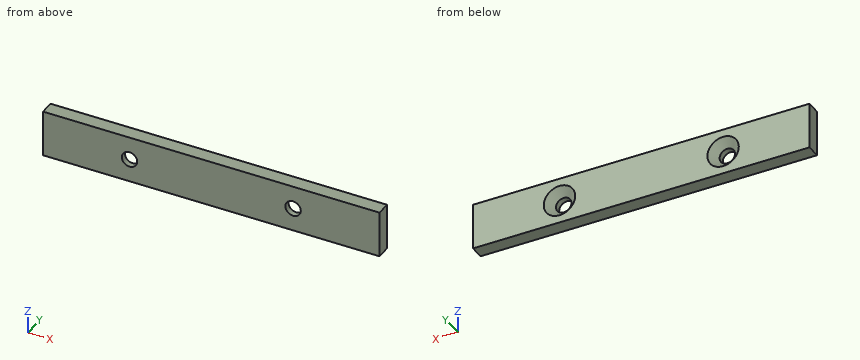
from build123d import *

# Parameters (mm, degrees)
SKETCH1_W                           = 144
SKETCH1_H                           = 20
EXTRUDE1_DEPTH                      = 6
ESCAREADO_PARA_SFHCS_M61_AT_2_COUNT = 2
ESCAREADO_PARA_SFHCS_M61_AT_2_PITCH = 70


with BuildPart() as part:
    # Sketch1 → Extrude1 (new body)
    with BuildSketch(Plane(origin=(0, 0, 0), x_dir=(1, 0, 0), z_dir=(0, 1, 0))):
        Rectangle(SKETCH1_W, SKETCH1_H)
    extrude(amount=EXTRUDE1_DEPTH)

    # Esboço1 → Escareado para SFHCS M61 (revolve, cut)
    with BuildSketch(Plane(origin=(-35, 6, 0), x_dir=(0, 0, 1), z_dir=(1, 0, 0))):
        Polygon((0, 0), (0, 6), (3.3, 6), (3.3, 3.42), (6.72, 0), align=None)
    escareado_para_sfhcs_m61 = revolve(axis=Axis((-35, 12.35, 0), (0, -1, 0)), mode=Mode.SUBTRACT)

    # Escareado para SFHCS M61 at 2: Escareado para SFHCS M61 ×2
    with Locations(*[(i * ESCAREADO_PARA_SFHCS_M61_AT_2_PITCH, 0, 0) for i in range(1, ESCAREADO_PARA_SFHCS_M61_AT_2_COUNT)]):
        add(escareado_para_sfhcs_m61, mode=Mode.SUBTRACT)


solid = part.part
Source: CAD feature listing. Evaluate the final solid. Frame: model axes, mm. Give positions to 0.01 mm unless a question says otherwise; leave off trailing zeros. Write each loop counter-clockwise with the first axis right and the second up, starting at its lowest first coordinate (ties: lowest second). Pieces come first, ordered by that corner, then holes. Notation, with made-up numbers: (-8, 6) -> (16, 6) arc R20 cw to (16, 12) -> close; hole circle Ø1 at (8, 10.5). An arc over 180 degrees is marked (long way). Return JSON: item names as keys, results as strings. Group by question number.
1. Section B-B, the plane z = 0. Output: boundary loops of the cut face in (x, y).
2. Material intervals for line 1 (X direction, y = 1.75, z = 0); line 2 (Z direction, x = -35, y = 1.35); line 3 (X direction, y = 2, z = -1), sorted ascending. Write a range as from..to.
3. Pin query (flat end, axial travel): pin 1 Ø6 at (x, z) = (35, 0) entering from +Y (3 decimals); pin 2 Ø10.5 at (x, z) = (-35, 0) entering from +Y. Return the tip coordinate at first contact, or that it passes through.
4. Section A-A, the plane x = -35. Output: boundary loops of the cut face in (y, z), then the cut area to 3 significant figures.
5. Section C-C, the plane y = 4.75. Output: boundary loops of the cut face in (x, z), then the cut area to 3 significant figures.
Determined:
{
 "1": {"outline": "(-72, 0) -> (-38.3, 0) -> (-38.3, 2.58) -> (-41.72, 6) -> (-72, 6) -> close; (-31.7, 0) -> (31.7, 0) -> (31.7, 2.58) -> (28.28, 6) -> (-28.28, 6) -> (-31.7, 2.58) -> close; (38.3, 0) -> (72, 0) -> (72, 6) -> (41.72, 6) -> (38.3, 2.58) -> close"},
 "2": {"line 1": "x = -72..-38.3, -31.7..31.7, 38.3..72", "line 2": "z = -10..-3.3, 3.3..10", "line 3": "x = -72..-38.14, -31.86..31.86, 38.14..72"},
 "3": {"pin 1": "passes through", "pin 2": "stops at y = 4.53"},
 "4": {"outline": "(0, -10) -> (6, -10) -> (6, -6.72) -> (2.58, -3.3) -> (0, -3.3) -> close; (0, 3.3) -> (2.58, 3.3) -> (6, 6.72) -> (6, 10) -> (0, 10) -> close", "area": "68.7 mm2"},
 "5": {"outline": "(-72, -10) -> (72, -10) -> (72, 10) -> (-72, 10) -> close; hole circle Ø10.94 at (-35, 0); hole circle Ø10.94 at (35, 0)", "area": "2,690 mm2"}
}
